Verification items for the finished model (mm, model axes). A direction names the side the tool comes from. Round coordinates to 2 decimals unless told otherwise and drop trailing zeros. Write each loop counter-clockwise with the first axis right and the second up, starting at its lowest first coordinate (ties: lowest second). Pieces come first, ordered by that corner, then holes. Notation, with made-up numbers: M 53,5.25 L 106,5.25 A33 ccw 106,37.25 Z; hole C 35.5,-28 d5. An arc over 180 degrees is marked long. Answer in a Markdown table with one row per item. Add a question column.
1. Go/stop test with flat-tipped pins: pin 1 Ø3 at (y, z) = (-3.5, 6.5) entering from -X; pin 2 Ø1 at (y, z) = (-6, 10) entering from -X; pin 3 Ø1.5 at (y, z) = (-1, 0.5) entering from +X. Record where each tip stops, or that it passes through.
2. Set-up check for faces 1 (the cylindrical face through (-6.094, 0.268, 6.261)), 2 (the flat face through (0, 0, 12.7)): record each of +Z, -Z, +X, -X, +Y, -Y from which the full face is reachable in a straight line by a thin tool's end or side.
3. Sectioned sample at C-C on z = 6.25. Record the cut outline in (x, y), plus the area to 3 significant figures.
4. Sectioned sample at D-D on z = -1.25. Record the cut outline in (x, y) (1 decimal).
5. Sectioned sample at A-A on x = 0. Record the cut outline in (y, z) (1 decimal), plus the area to 3 significant figures.
6. Material ranges on probe 1 along Y at (x, z) = (0, 6); probe 2 along Z at (x, y) = (-6, -2.25) (3 decimals); probe 3 along X at (y, z) = (0.25, 9.5), recorded low to high.
```python
from build123d import *

# Parameters (mm, degrees)
SKETCH1_R           = 6.35
BOSS_EXTRUDE1_DEPTH = 12.7
SKETCH2_R           = 7.9375
BOSS_EXTRUDE2_DEPTH = 3.175
MOVE_FACE1_BY       = 0.25


with BuildPart() as part:
    # Sketch1 → Boss-Extrude1 (new body)
    with BuildSketch(Plane.XY):
        Circle(SKETCH1_R)
    extrude(amount=BOSS_EXTRUDE1_DEPTH)

    # Sketch2 → Boss-Extrude2 (add)
    with BuildSketch(Plane(origin=(0, 0, 0), x_dir=(-1, 0, 0), z_dir=(0, 0, -1))):
        Circle(SKETCH2_R)
    extrude(amount=BOSS_EXTRUDE2_DEPTH)

    # Move Face1: a curved face moved inward by 0.25
    add(Solid.thicken(part.faces().sort_by_distance((-6.35, 0, 6.35))[0], -MOVE_FACE1_BY), mode=Mode.SUBTRACT)


solid = part.part
```
Geometry check:
| question | item | result |
|---|---|---|
| 1 | pin 1 | stops at x = -5.76 |
| 1 | pin 2 | stops at x = -2.64 |
| 1 | pin 3 | stops at x = 7.93 |
| 2 | face 1 | +Z |
| 2 | face 2 | +Z, +X, -X, +Y, -Y |
| 3 | outline | C 0,0 d12.2 |
| 3 | area | 117 mm2 |
| 4 | outline | C 0,0 d15.9 |
| 5 | outline | M -7.9,-3.2 L 7.9,-3.2 L 7.9,0 L 6.1,0 L 6.1,12.7 L -6.1,12.7 L -6.1,0 L -7.9,0 Z |
| 5 | area | 205 mm2 |
| 6 | probe 1 | y = -6.1 to 6.1 |
| 6 | probe 2 | z = -3.175 to 0 |
| 6 | probe 3 | x = -6.09 to 6.09 |
